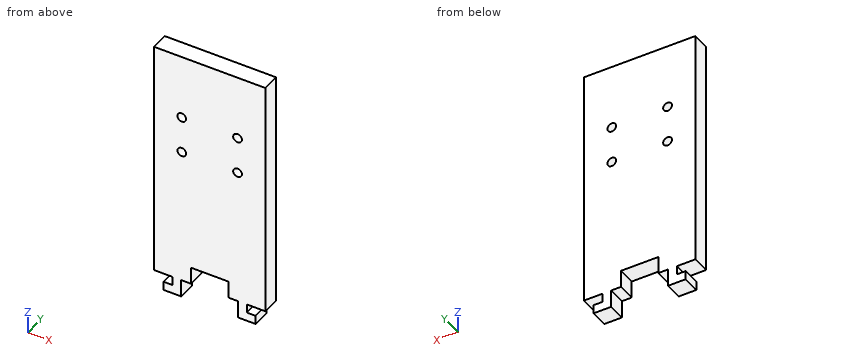
from build123d import *

# Parameters (mm, degrees)
BOSS_EXTRUDE1_DEPTH     = 2.999999969
CUT_EXTRUDE1_DEPTH      = 54.841456961
CUT_EXTRUDE1_DEPTH_BACK = 54.841456961
SKETCH2_R               = 1.5


with BuildPart() as part:
    # Sketch1 → Boss-Extrude1 (new, symmetric)
    with BuildSketch(Plane(origin=(0, 0, 0), x_dir=(1, 0, 0), z_dir=(0, 1, 0))):
        Polygon((15.7, 43.999999884), (12.7, 43.999999884), (9.7, 43.999999884), (6.35, 43.999999884), (6.35, 38.1), (-6.35, 38.1), (-6.35, 43.999999884), (-9.7, 43.999999884), (-12.7, 43.999999884), (-15.7, 43.999999884), (-19.05, 43.999999884), (-19.05, 38.1), (-19.05, -38.1), (19.05, -38.1), (19.05, 38.1), (19.05, 43.999999884), align=None)
        Polygon((-12.7, 43.999999884), (-9.7, 43.999999884), (-9.7, 49.999999884), (-15.7, 49.999999884), (-15.7, 46.999999884), (-12.7, 46.999999884), align=None)
        Polygon((9.7, 43.999999884), (12.7, 43.999999884), (12.7, 46.999999884), (15.7, 46.999999884), (15.7, 49.999999884), (9.7, 49.999999884), align=None)
    extrude(amount=BOSS_EXTRUDE1_DEPTH, both=True)

    # Sketch2 → Cut-Extrude1 (cut, two sides: drawn at the far end of the back side and taken through both)
    with BuildSketch(Plane(origin=(0, 2.999999969, 0), x_dir=(1, 0, 0), z_dir=(0, 1, 0)).offset(-CUT_EXTRUDE1_DEPTH_BACK)):
        with Locations(Location((-9.525, -3.175, 0), (0, 0, 270))):
            Circle(SKETCH2_R)
        with Locations(Location((9.525, -3.175, 0), (0, 0, 270))):
            Circle(SKETCH2_R)
        with Locations(Location((9.525, -15.875, 0), (0, 0, 270))):
            Circle(SKETCH2_R)
        with Locations(Location((-9.525, -15.875, 0), (0, 0, 270))):
            Circle(SKETCH2_R)
    extrude(amount=CUT_EXTRUDE1_DEPTH + CUT_EXTRUDE1_DEPTH_BACK, mode=Mode.SUBTRACT)


solid = part.part
Can you work these out from the model? Positions are in its coordinate system, mm. Give positions to 0.01 mm unless a question says otherwise; leave off trailing zeros. Loops run counter-clockwise (first coordinate to the right, second up) from the corner with the lowest first, then second, coordinate; pieces in that order, holes last. Notation, with made-up numbers: (79, -33.75) -> (118, -33.75) arc R26 ccw to (118, -13.75) -> close; hole circle Ø1 at (6.5, 24). An arc over 180 degrees is marked (long way). Use one line per item in the form item = value.
1) If we section it at B-B (y = 1.35): Please give me the cut outline in (x, z) (3 decimals).
Answers:
outline = (-19.05, -44) -> (-12.7, -44) -> (-12.7, -47) -> (-15.7, -47) -> (-15.7, -50) -> (-9.7, -50) -> (-9.7, -44) -> (-6.35, -44) -> (-6.35, -38.1) -> (6.35, -38.1) -> (6.35, -44) -> (9.7, -44) -> (9.7, -50) -> (15.7, -50) -> (15.7, -47) -> (12.7, -47) -> (12.7, -44) -> (19.05, -44) -> (19.05, 38.1) -> (-19.05, 38.1) -> close; hole circle Ø3 at (-9.525, 3.175); hole circle Ø3 at (-9.525, 15.875); hole circle Ø3 at (9.525, 3.175); hole circle Ø3 at (9.525, 15.875)
2) If we section it at C-C (x = 1): Please give me the cut outline in (y, z), plus the area to 3 significant figures.
Answers:
outline = (-3, -38.1) -> (3, -38.1) -> (3, 38.1) -> (-3, 38.1) -> close
area = 457 mm²
3) Will these pins go through, and if not, where does the flat tip stop? pin 1 (0.9 mm diameter, centred on y = 0, z = -46, fed in from +X); pin 2 (2.5 mm diameter, centred on x = 9.525, z = 15.875, fed in from +Y); pin 3 (3.5 mm diameter, centred on y = -1.5, z = -48.5, fed in from -X); pin 4 (1 mm diameter, centred on x = 8, y = 1.5, fed in from -Z).
Answers:
pin_1 = 12.7
pin_2 = through
pin_3 = -15.7
pin_4 = -44
4) I need wall thicknesses on line 1 along X through (y, z) = (-0.75, 3); line 2 along X through (y, z) = (-1.75, -41); line 3 along Z through (x, y) = (9, 0.3). Which ranges of each line are inside material? Lowest first, please.
Answers:
line_1 = -19.05 to -11.01, -8.04 to 8.04, 11.01 to 19.05
line_2 = -19.05 to -6.35, 6.35 to 19.05
line_3 = -44 to 1.77, 4.58 to 14.47, 17.28 to 38.1
5) If we section it at A-A (z = -40): Please give me the cut outline in (x, y), plus the area to 3 significant figures.
Answers:
outline = (-19.05, -3) -> (-6.35, -3) -> (-6.35, 3) -> (-19.05, 3) -> close; (6.35, -3) -> (19.05, -3) -> (19.05, 3) -> (6.35, 3) -> close
area = 152 mm²
